Check sheet for the drawn part. Datum: minimum x, y, z corner. Units: mm. A direction names the side the tool comes from. Round coordinates to 2 decimals unless told otherwise and drop trailing zeros. Write each loop counter-clockwise with the first axis right and the second up, starting at its lowest first coordinate (ties: lowest second). Pieces come first, ordered by that corner, then holes. Notation, with made-up numbers: M -21,29.25 L 16,29.25 A20 cw 16,55.25 Z; hole C -26.75,-10.75 d1. An arc over 180 degrees is marked long. Use a Markdown table: item, result.
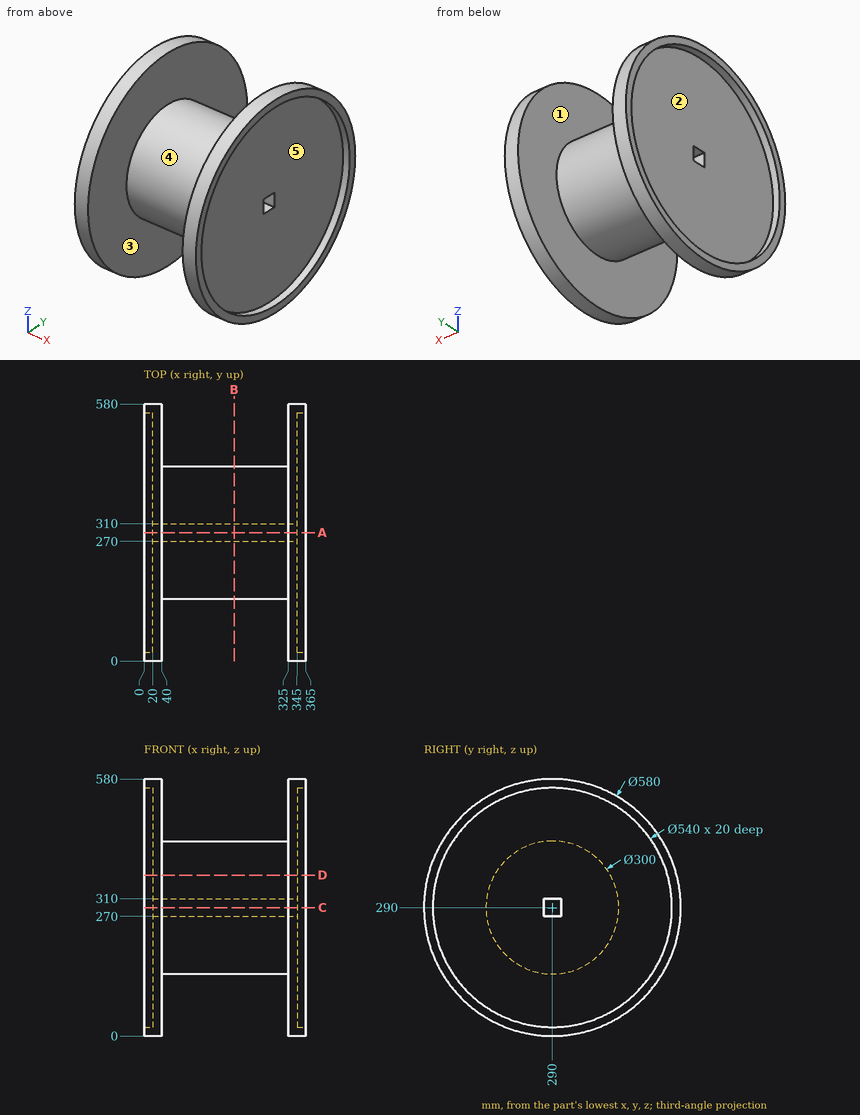
Item 1: Cross-section at B-B, the plane x = 203. Record the cut outline in (y, z), and give its area (3 significant figures).
Outcome:
| item | result |
|---|---|
| outline | C 290,290 d300; hole M 270,270 L 310,270 L 310,310 L 270,310 Z |
| area | 69,100 mm2 |
Item 2: Material ranges on line 1 along X through (y, z) = (41, 161); line 2 along Y through (x, z) = (350.75, 290); line 3 along X through (y, z) = (468.5, 473), recorded low to high. Write a range as from..to.
Outcome:
| item | result |
|---|---|
| line 1 | x = 0..40, 325..365 |
| line 2 | y = 0..20, 560..580 |
| line 3 | x = 20..40, 325..345 |
Item 3: Access from +Z, -Z, +X, -X, +Y, -Y to the whole of each face (thin tool, end or side, straight path). Record for the marked faces 1 and 2.
Outcome:
| item | result |
|---|---|
| face 1 | none |
| face 2 | -X |
Item 4: Cross-section at A-A, the plane y = 290. Record the cut outline in (x, z).
Outcome:
| item | result |
|---|---|
| outline | M 0,0 L 40,0 L 40,140 L 325,140 L 325,0 L 365,0 L 365,20 L 345,20 L 345,270 L 20,270 L 20,20 L 0,20 Z; M 0,560 L 20,560 L 20,310 L 345,310 L 345,560 L 365,560 L 365,580 L 325,580 L 325,440 L 40,440 L 40,580 L 0,580 Z |
Item 5: Cross-section at D-D, the plane z = 363. Record the cut outline in (x, y), and give its area (3 significant figures).
Outcome:
| item | result |
|---|---|
| outline | M 0,9.34 L 40,9.34 L 40,158.96 L 325,158.96 L 325,9.34 L 365,9.34 L 365,30.06 L 345,30.06 L 345,549.94 L 365,549.94 L 365,570.66 L 325,570.66 L 325,421.04 L 40,421.04 L 40,570.66 L 0,570.66 L 0,549.94 L 20,549.94 L 20,30.06 L 0,30.06 Z |
| area | 98,800 mm2 |
Item 6: Mould release check, pull along Y, two halves, no side actions. Record for the marked faces 3, 4 and 5: +Y half, -Y half, draft (parallel to the pull), parting line (faces both ways), or undercut.
Outcome:
| item | result |
|---|---|
| face 3 | draft |
| face 4 | parting line |
| face 5 | undercut |
Item 7: Go/stop test with flat-tipped pins: pin 1 (2 mm diameter, centred on y = 370, z = 430.5, fed in from -X); pin 2 (12 mm diameter, centred on x = 236, y = 294.5, fed in from -Z); pin 3 (8 mm diameter, centred on x = 328, y = 434.5, fed in from +Z). Record where each tip stops, or that it passes through.
Outcome:
| item | result |
|---|---|
| pin 1 | stops at x = 20 |
| pin 2 | stops at z = 140 |
| pin 3 | stops at z = 543.69 |
